Here's how the part is built. I have some questions about the finished solid (model axes, mm). A direction names the side the tool comes from. Round coordinates to 2 decimals unless told otherwise and drop trailing zeros. Loops run counter-clockwise (first coordinate to the right, second up) from the corner with the lowest first, then second, coordinate; pieces in that order, holes last. Notation, with made-up numbers: M 49,82 L 93,82 A22 cw 93,109 Z; hole C 5.25,24 d5. An arc over 180 degrees is marked long. Use a Markdown table: item, result.
```python
from build123d import *

# Parameters (mm, degrees)
SKETCH1_W           = 55
SKETCH1_H           = 30
BOSS_EXTRUDE2_DEPTH = 2
SKETCH8_W           = 27
SKETCH8_H           = 23
SKETCH8_W_2         = 21
SKETCH8_H_2         = 17
BOSS_EXTRUDE3_DEPTH = 10
SKETCH10_W          = 21
SKETCH10_H          = 14
BOSS_EXTRUDE4_DEPTH = 2
SKETCH13_W          = 21
SKETCH13_H          = 5
CUT_EXTRUDE3_DEPTH  = 3
SKETCH14_R          = 1.5
BOSS_EXTRUDE5_DEPTH = 3


with BuildPart() as part:
    # Sketch1 → Boss-Extrude2 (new body)
    with BuildSketch(Plane.XY):
        Rectangle(SKETCH1_W, SKETCH1_H)
    extrude(amount=BOSS_EXTRUDE2_DEPTH)

    # Sketch8 → Boss-Extrude3 (add)
    with BuildSketch(Plane.XY.offset(2)):
        Rectangle(SKETCH8_W, SKETCH8_H)
        Rectangle(SKETCH8_W_2, SKETCH8_H_2, mode=Mode.SUBTRACT)
    extrude(amount=BOSS_EXTRUDE3_DEPTH)

    # Sketch10 → Boss-Extrude4 (add)
    with BuildSketch(Plane.XY.offset(2)):
        with Locations((0, 1.5)):
            Rectangle(SKETCH10_W, SKETCH10_H)
    extrude(amount=BOSS_EXTRUDE4_DEPTH)

    # Sketch13 → Cut-Extrude3 (cut)
    with BuildSketch(Plane.XZ.offset(11.5)):
        with Locations((0, 9.5)):
            Rectangle(SKETCH13_W, SKETCH13_H)
    extrude(amount=-CUT_EXTRUDE3_DEPTH, mode=Mode.SUBTRACT)

    # Sketch14 → Boss-Extrude5 (add)
    with BuildSketch(Plane.XY.offset(4)):
        with Locations((-8, 6)):
            Circle(SKETCH14_R)
        with Locations((8, 6)):
            Circle(SKETCH14_R)
    extrude(amount=BOSS_EXTRUDE5_DEPTH)


solid = part.part
```
Q1. We'd pull the mould along Y, two halves only. Please class faces 6 (the flat face through (-8, 6, 7)), 7 (the flat face through (0, 2, 4)), 8 (the flat face through (0, 15, 1)): pulls with the +Y half, pulls with the -Y half, needs draft (parallel to the pull), parting line crosses it, or undercut.
Return value:
| item | result |
|---|---|
| face 6 | needs draft |
| face 7 | undercut |
| face 8 | pulls with the +Y half |
Q2. Imagine slicing it at D-D, the plane z = 11. Please give me the cut outline in (x, y), then the cut area to 3 significant figures.
Return value:
| item | result |
|---|---|
| outline | M -13.5,-11.5 L -10.5,-11.5 L -10.5,8.5 L 10.5,8.5 L 10.5,-11.5 L 13.5,-11.5 L 13.5,11.5 L -13.5,11.5 Z |
| area | 201 mm^2 |
Q3. Imagine slicing it at C-C, the plane x = -8. Please give me the cut outline in (y, z).
Return value:
| item | result |
|---|---|
| outline | M -15,0 L 15,0 L 15,2 L 11.5,2 L 11.5,12 L 8.5,12 L 8.5,4 L 7.5,4 L 7.5,7 L 4.5,7 L 4.5,4 L -5.5,4 L -5.5,2 L -8.5,2 L -8.5,7 L -11.5,7 L -11.5,2 L -15,2 Z |
Q4. Imagine slicing it at A-A, the plane z = 6. Please give me the cut outline in (x, y), then the cut area to 3 significant figures.
Return value:
| item | result |
|---|---|
| outline | M -13.5,-11.5 L 13.5,-11.5 L 13.5,11.5 L -13.5,11.5 Z; C -8,6 d3; C 8,6 d3; hole M -10.5,-8.5 L 10.5,-8.5 L 10.5,8.5 L -10.5,8.5 Z |
| area | 278 mm^2 |
Q5. I need wall thicknesses on line 1 (X direction, y = 1.5, z = 8); line 2 (Y direction, x = 3.5, z = 6); line 3 (X direction, y = 8.25, z = 2.75). Which ranges of each line are inside material? Lowest first, please. Write a range as from..to.
Return value:
| item | result |
|---|---|
| line 1 | x = -13.5..-10.5, 10.5..13.5 |
| line 2 | y = -11.5..-8.5, 8.5..11.5 |
| line 3 | x = -13.5..13.5 |
Q6. Will these pins go through, and if not, where does the flat tip stop? P1, Ø4, axis at x = -7.5, z = 6.5, coming from the -Y side; P2, Ø0.9, axis at x = 4, y = -7, coming from the +Z side; P3, Ø5, axis at y = 1.5, z = 6.5, coming from the -X side.
Return value:
| item | result |
|---|---|
| P1 | stops at y = -11.5 |
| P2 | stops at z = 2 |
| P3 | stops at x = -13.5 |
Q7. For faces 1 (the flat face through (-13.5, 0, 7)), 2 (the flat face through (8, 6, 7)), 3 (the flat face through (0, -11.5, 6)), 4 (the flat face through (0, -8.5, 4)), 5 (the flat face through (0, 11.5, 7)), which set-ups out of +Z, -Z, +X, -X, +Y, -Y let a thin tool reach every point of the face, with its end or its side?
Return value:
| item | result |
|---|---|
| face 1 | +Z, -X, +Y, -Y |
| face 2 | +Z, -Y |
| face 3 | +Z, +X, -X, -Y |
| face 4 | +Z |
| face 5 | +Z, +X, -X, +Y |
Q8. Imagine slicing it at B-B, the plane y = 6. Please give me the cut outline in (x, z), then the cut area to 3 significant figures.
Return value:
| item | result |
|---|---|
| outline | M -27.5,0 L 27.5,0 L 27.5,2 L 13.5,2 L 13.5,12 L 10.5,12 L 10.5,4 L 9.5,4 L 9.5,7 L 6.5,7 L 6.5,4 L -6.5,4 L -6.5,7 L -9.5,7 L -9.5,4 L -10.5,4 L -10.5,12 L -13.5,12 L -13.5,2 L -27.5,2 Z |
| area | 230 mm^2 |
